from build123d import *

# Parameters (mm, degrees)
EXTRUDE_1_DEPTH               = 12.5
EXTRUDE_1_DEPTH_BACK          = 12.5
SKETCH_1_W                    = 25
SKETCH_1_H                    = 4.5
CUT_EXTRUDE_1_DEPTH           = 0.2
CUT_EXTRUDE_1_DEPTH_BACK      = 0.2
PATTERN_LINEAR_1_COUNT        = 2
PATTERN_LINEAR_1_PITCH        = 20
PATTERN_LINEAR_1_COUNT_DIR2   = 2
PATTERN_LINEAR_1_PITCH_DIR2   = 20
EXTRUDE_2_DEPTH               = 3.5
SKETCH_8_W                    = 25
SKETCH_8_H                    = 4
EXTRUDE_3_DEPTH               = 2
EXTRUDE_4_DEPTH               = 4.2
SKETCH_10_R                   = 3
CUT_EXTRUDE_2_DEPTH           = 4.2
EXTRUDE_5_DEPTH               = 4.2
SKETCH_12_R                   = 4
CUT_EXTRUDE_3_DEPTH           = 4.2
SKETCH_13_W                   = 2
SKETCH_13_H                   = 1.9
CUT_EXTRUDE_4_DEPTH           = 1
SKETCH_15_R                   = 4
CUT_EXTRUDE_5_DEPTH           = 1
SKETCH_16_W                   = 2
SKETCH_16_H                   = 1.9
CUT_EXTRUDE_6_DEPTH           = 1
EXTRUDE_START                 = 9.5
EXTRUDE_6_DEPTH               = 9.5
CUT_REVOLVE_2_ANGLE           = 50
CUT_REVOLVE_2_OTHER_WAY_ANGLE = 50
CUT_EXTRUDE_7_DEPTH           = 0.5
SKETCH_22_R                   = 1.5
CUT_EXTRUDE_8_DEPTH           = 8.5


with BuildPart() as part:
    # Sketch 1 → Extrude 1 (new, two sides: drawn at the far end of the back side and taken through both)
    with BuildSketch(Plane.XY.offset(-EXTRUDE_1_DEPTH_BACK)):
        with Locations((0, 2.25)):
            Rectangle(SKETCH_1_W, SKETCH_1_H)
    extrude(amount=EXTRUDE_1_DEPTH + EXTRUDE_1_DEPTH_BACK)

    # Sketch 2 → Revolve 1 (revolve)
    with BuildSketch(Plane(origin=(0, 0, 0), x_dir=(0, 0, -1), z_dir=(1, 0, 0))):
        Polygon((0, 4.5), (-12, 4.5), (-12, 8.5), (-11, 8.5), (-11, 5.5), (0, 5.5), align=None)
    revolve(axis=Axis((0, 5.5, 0), (0, -1, 0)))

    # Sketch 3 → Cut-Extrude 1 (cut, two sides: drawn at the far end of the back side and taken through both)
    with BuildSketch(Plane(origin=(0, 0, 0), x_dir=(1, 0, 0), z_dir=(0, 1, 0)).offset(-CUT_EXTRUDE_1_DEPTH_BACK)):
        Polygon((-12.5, 4.5), (-12.5, -4.5), (-4.5, -4.5), (-4.5, -12.5), (4.5, -12.5), (4.5, -4.5), (12.5, -4.5), (12.5, 4.5), (4.5, 4.5), (4.5, 12.5), (-4.5, 12.5), (-4.5, 4.5), align=None)
    extrude(amount=CUT_EXTRUDE_1_DEPTH + CUT_EXTRUDE_1_DEPTH_BACK, mode=Mode.SUBTRACT)

    # Sketch 4 → Cut-Revolve 1 (revolve, cut)
    with BuildSketch(Plane(origin=(-10, 0, 0), x_dir=(0, 0, -1), z_dir=(1, 0, 0))):
        Polygon((10, 0), (8.75, 0), (8.75, 2), (7.9, 2), (7.9, 4.5), (10, 4.5), align=None)
    cut_revolve_1 = revolve(axis=Axis((-10, 4.5, -10), (0, -1, 0)), mode=Mode.SUBTRACT)

    # Pattern Linear 1: Cut-Revolve 1 2 × 2
    with Locations(*[(i * PATTERN_LINEAR_1_PITCH, 0, j * PATTERN_LINEAR_1_PITCH_DIR2) for i in range(PATTERN_LINEAR_1_COUNT) for j in range(PATTERN_LINEAR_1_COUNT_DIR2) if (i, j) != (0, 0)]):
        add(cut_revolve_1, mode=Mode.SUBTRACT)

    # Sketch 6 → Extrude 2 (add)
    with BuildSketch(Plane(origin=(0, 4.5, 0), x_dir=(1, 0, 0), z_dir=(0, 1, 0))):
        with BuildLine():
            Line((11.363205929, 3.857142857), (11.363205929, -3.857142857))
            ThreePointArc((11.363205929, -3.857142857), (12.092108839, -2.874313332), (13.257073584, -2.5))
            Line((13.257073584, -2.5), (22, -2.5))
            Line((22, -2.5), (22, 2.5))
            Line((22, 2.5), (13.257073584, 2.5))
            ThreePointArc((13.257073584, 2.5), (12.092108839, 2.874313332), (11.363205929, 3.857142857))
        make_face()
    extrude(amount=EXTRUDE_2_DEPTH)

    # Sketch 7 → Revolve 2 (revolve)
    with BuildSketch(Plane.XY, mode=Mode.PRIVATE) as revolve_2_sk:
        Polygon((21.9, 6.2), (21.9, 7.7), (22.5, 7.7), (22.5, 8.2), (23.5, 8.2), (23.5, 9.2), (26.2, 9.2), (26.7, 8.7), (26.7, 6.2), align=None)
    revolve(revolve_2_sk.sketch.rotate(Axis((26.7, 6.2, 0), (-1, 0, 0)), 270), axis=Axis((26.7, 6.2, 0), (-1, 0, 0)))

    # Sketch 8 → Extrude 3 (add)
    with BuildSketch(Plane(origin=(12.5, 0, 0), x_dir=(0, 0, -1), z_dir=(1, 0, 0))):
        with Locations((0, 2.2)):
            Rectangle(SKETCH_8_W, SKETCH_8_H)
    extrude(amount=EXTRUDE_3_DEPTH)

    # Sketch 9 → Extrude 4 (add)
    with BuildSketch(Plane.XY.offset(12.5)):
        Polygon((13, 0.2), (22.5, 0.2), (23.5, 1.2), (23.5, 10.2), (22.5, 11.2), (13, 11.2), align=None)
    extrude(amount=-EXTRUDE_4_DEPTH)

    # Sketch 10 → Cut-Extrude 2 (cut)
    with BuildSketch(Plane.XY.offset(12.5)):
        with Locations((19, 6.5)):
            Circle(SKETCH_10_R)
    extrude(amount=-CUT_EXTRUDE_2_DEPTH, mode=Mode.SUBTRACT)

    # Sketch 11 → Extrude 5 (add)
    with BuildSketch(Plane.XY.offset(-12.5)):
        Polygon((13, 0.2), (22.5, 0.2), (23.5, 1.2), (23.5, 10.2), (22.5, 11.2), (13, 11.2), align=None)
    extrude(amount=EXTRUDE_5_DEPTH)

    # Sketch 12 → Cut-Extrude 3 (cut)
    with BuildSketch(Plane.XY.offset(-12.5)):
        with Locations((19, 6.5)):
            Circle(SKETCH_12_R)
    extrude(amount=CUT_EXTRUDE_3_DEPTH, mode=Mode.SUBTRACT)

    # Sketch 13 → Revolve 3 (revolve)
    with BuildSketch(Plane.XY.offset(-3), mode=Mode.PRIVATE) as revolve_3_sk:
        with Locations((15.5, 3.45)):
            Rectangle(SKETCH_13_W, SKETCH_13_H)
    revolve(revolve_3_sk.sketch.rotate(Axis((16.5, 2.5, -3), (-1, 0, 0)), 270), axis=Axis((16.5, 2.5, -3), (-1, 0, 0)))

    # Sketch 14 → Cut-Extrude 4 (cut)
    with BuildSketch(Plane(origin=(16.5, 0, 0), x_dir=(0, 0, -1), z_dir=(1, 0, 0))):
        Polygon((2.566987298, 1.75), (3.433012702, 1.75), (3.866025404, 2.5), (3.433012702, 3.25), (2.566987298, 3.25), (2.133974596, 2.5), align=None)
    extrude(amount=-CUT_EXTRUDE_4_DEPTH, mode=Mode.SUBTRACT)

    # Sketch 15 → Cut-Extrude 5 (cut)
    with BuildSketch(Plane.XY.offset(8.3)):
        with Locations((19, 6.2)):
            Circle(SKETCH_15_R)
    extrude(amount=CUT_EXTRUDE_5_DEPTH, mode=Mode.SUBTRACT)

    # Sketch 16 → Revolve 4 (revolve)
    with BuildSketch(Plane.XY.offset(3), mode=Mode.PRIVATE) as revolve_4_sk:
        with Locations((15.5, 3.45)):
            Rectangle(SKETCH_16_W, SKETCH_16_H)
    revolve(revolve_4_sk.sketch.rotate(Axis((16.5, 2.5, 3), (-1, 0, 0)), 270), axis=Axis((16.5, 2.5, 3), (-1, 0, 0)))

    # Sketch 17 → Cut-Extrude 6 (cut)
    with BuildSketch(Plane(origin=(16.5, 0, 0), x_dir=(0, 0, -1), z_dir=(1, 0, 0))):
        Polygon((-3.433012702, 1.75), (-2.566987298, 1.75), (-2.133974596, 2.5), (-2.566987298, 3.25), (-3.433012702, 3.25), (-3.866025404, 2.5), align=None)
    extrude(amount=-CUT_EXTRUDE_6_DEPTH, mode=Mode.SUBTRACT)

    # Sketch 18 → Extrude 6 (add)
    with BuildSketch(Plane(origin=(0, 0, 0), x_dir=(1, 0, 0), z_dir=(0, 1, 0)).offset(EXTRUDE_START)):
        with BuildLine():
            Line((5, -13.610657589), (5, -10.908712115))
            ThreePointArc((5, -10.908712115), (0, -12), (-5, -10.908712115))
            Line((-5, -10.908712115), (-5, -13.610657589))
            ThreePointArc((-5, -13.610657589), (0, -14.5), (5, -13.610657589))
        make_face()
    extrude(amount=-EXTRUDE_6_DEPTH)

    # Sketch 19 → Cut-Revolve 2 (revolve, cut)
    with BuildSketch(Plane(origin=(0, 0, 0), x_dir=(0, 0, -1), z_dir=(1, 0, 0))):
        Polygon((-16, 4.5), (-15, 4.5), (-13.606664199, 9.7), (-16, 9.7), align=None)
    revolve(axis=Axis((0, 9.7, 0), (0, -1, 0)), revolution_arc=CUT_REVOLVE_2_ANGLE, mode=Mode.SUBTRACT)

    # Sketch 19 → Cut-Revolve 2 other way (revolve, cut)
    with BuildSketch(Plane(origin=(0, 0, 0), x_dir=(0, 0, -1), z_dir=(1, 0, 0))):
        Polygon((-16, 4.5), (-15, 4.5), (-13.606664199, 9.7), (-16, 9.7), align=None)
    revolve(axis=Axis((0, 9.7, 0), (0, 1, 0)), revolution_arc=CUT_REVOLVE_2_OTHER_WAY_ANGLE, mode=Mode.SUBTRACT)

    # Sketch 20 → Revolve 5 (revolve)
    with BuildSketch(Plane(origin=(0, 0, 0), x_dir=(0, 0, -1), z_dir=(1, 0, 0)), mode=Mode.PRIVATE) as revolve_5_sk:
        Polygon((-14, 2), (-14, 1), (-15.3, 1), (-15.5, 1.2), (-15.5, 2), align=None)
    revolve(revolve_5_sk.sketch.rotate(Axis((0, 2, 15.5), (0, 0, -1)), 270), axis=Axis((0, 2, 15.5), (0, 0, -1)))

    # Sketch 21 → Cut-Extrude 7 (cut)
    with BuildSketch(Plane.XY.offset(15.5)):
        Polygon((0.15, 2.5), (-0.15, 2.5), (-0.15, 2.15), (-0.5, 2.15), (-0.5, 1.85), (-0.15, 1.85), (-0.15, 1.5), (0.15, 1.5), (0.15, 1.85), (0.5, 1.85), (0.5, 2.15), (0.15, 2.15), align=None)
    extrude(amount=-CUT_EXTRUDE_7_DEPTH, mode=Mode.SUBTRACT)

    # Sketch 22 → Cut-Extrude 8 (cut)
    with BuildSketch(Plane(origin=(0, 0, 0), x_dir=(1, 0, 0), z_dir=(0, 1, 0))):
        with Locations(Location((0, 0, 0), (0, 0, 270))):
            Circle(SKETCH_22_R)
    extrude(amount=CUT_EXTRUDE_8_DEPTH, mode=Mode.SUBTRACT)


solid = part.part
Work out the finished part from the listing and answer in its coordinate system (mm). A direction names the side the tool comes from. Round coordinates to 2 decimals unless told otherwise and drop trailing zeros. Write each loop counter-clockwise with the first axis right and the second up, starting at its lowest first coordinate (ties: lowest second). Pieces come first, ordered by that corner, then holes.
1) Straight lines are drawn through the part: line 1 (Z direction, x = -10, y = 2.9); line 2 (Z direction, x = -10, y = 1.4); line 3 (X direction, y = 1.3, z = 10). For each, find the intervals that lie inside material, in ascending order.
2) A cutting plane is placed at D-D (z = -5.5). Give the vertices of the cut face in (x, y).
3) Given pin 1 Ø1.5 at (x, y) = (17.5, 2) entering from +Z; pin 2 Ø2 at (x, z) = (-10, -10.5) entering from +Y; pin 3 Ø8 at (x, z) = (19.5, 5) entering from +Y; pin 4 Ø5 at (x, z) = (6, 3) entering from +Y, each flat-ended and moving along its own axis, determine where each tip first touches the part or whether it passes through.
4) The mould has two halves that part along Y. Classify faces 5 (the conical face through (-0.074, 7.955, 14.074)), 6 (the flat face through (22, 7.39, 1.15)), 7 (the flat face through (16, 3.25, -3)): pulls with the +Y half, pulls with the -Y half, needs draft (parallel to the pull), parting line crosses it, or undercut.
5) A tool of negligible diameter and unlimited length cuts with its end or side. For faces 1 (the flat face through (18, 6, -2.5)), 2 (the flat face through (16, 4, 12.5)), 3 (the flat face through (13, 8, -10)), 4 (the flat face through (23.5, 4, -1)), from which of +Z, -Z, +X, -X, +Y, -Y can it reach the whole face along a straight path? Write none if from no direction.
6) A cutting plane is placed at B-B (x = -10). Give the number of separate pieces and of enclosed holes in the cut face, plus the area to 3 significant figures.
Completed:
1. line 1: z = -12.5 to -12.1, -7.9 to 7.9, 12.1 to 12.5
1. line 2: z = -12.5 to -11.25, -8.75 to 8.75, 11.25 to 12.5
1. line 3: x = -12.5 to -11.25, -8.75 to 8.75, 11.25 to 23.5
2. outline: (-12.5, 0) - (-4.5, 0) - (-4.5, 0.2) - (4.5, 0.2) - (4.5, 0) - (12.5, 0) - (12.5, 0.2) - (14.5, 0.2) - (14.5, 4.2) - (12.5, 4.2) - (12.5, 4.5) - (10.67, 4.5) - (10.67, 8.5) - (9.53, 8.5) - (9.53, 5.5) - (-9.53, 5.5) - (-9.53, 8.5) - (-10.67, 8.5) - (-10.67, 4.5) - (-12.5, 4.5) - close
3. pin 1: stops at z = 12.5
3. pin 2: stops at y = 2
3. pin 3: stops at y = 11.2
3. pin 4: stops at y = 5.5
4. face 5: pulls with the +Y half
4. face 6: needs draft
4. face 7: undercut
5. face 1: +Y
5. face 2: +Z, +X, +Y, -Y
5. face 3: -Z, +Y
5. face 4: none
6. separate pieces: 3
6. enclosed holes: 0
6. area: 105 mm2
